Check sheet for the modelled part. Datum: model origin and axes. Units: mm. A direction names the side the tool comes from. Give positions to 0.01 mm unless a question says otherwise; leave off trailing zeros. Write each loop counter-clockwise with the first axis right and the second up, starting at its lowest first coordinate (ties: lowest second). Pieces come first, ordered by that corner, then holes. Notation, with made-up numbers: (6, -26.5) -> (33, -26.5) arc R14 cw to (33, -9.5) -> close; hole circle Ø8 at (22, 56). An arc over 180 degrees is marked (long way). Return JSON: item names as keys, results as strings.
from build123d import *

# Parameters (mm, degrees)
SKETCH1_W           = 72
SKETCH1_H           = 47
BOSS_EXTRUDE1_DEPTH = 4
SKETCH3_W           = 72
SKETCH3_H           = 47
SKETCH3_W_2         = 67
SKETCH3_H_2         = 42
BOSS_EXTRUDE3_DEPTH = 26
SKETCH5_W           = 12
SKETCH5_H           = 8
CUT_EXTRUDE1_DEPTH  = 6
FILLET2_R           = 2
FILLET3_R           = 2
SKETCH11_W          = 24
SKETCH11_H          = 20
BOSS_EXTRUDE7_DEPTH = 20
SKETCH12_W          = 20
SKETCH12_H          = 16
CUT_EXTRUDE4_DEPTH  = 20
SKETCH13_W          = 15
SKETCH13_H          = 9
CUT_EXTRUDE5_DEPTH  = 20
FILLET4_R           = 2
FILLET5_R           = 2
SKETCH14_W          = 6
SKETCH14_H          = 25
CUT_EXTRUDE6_DEPTH  = 5
FILLET6_R           = 2
SKETCH15_W          = 68
SKETCH15_H          = 6
BOSS_EXTRUDE8_DEPTH = 25
FILLET7_R           = 5
CUT_EXTRUDE7_DEPTH  = 25


with BuildPart() as part:
    # Sketch1 → Boss-Extrude1 (new body)
    with BuildSketch(Plane(origin=(0, 0, 0), x_dir=(1, 0, 0), z_dir=(0, 1, 0))):
        with Locations((25.5, 13)):
            Rectangle(SKETCH1_W, SKETCH1_H)
    extrude(amount=BOSS_EXTRUDE1_DEPTH)

    # Sketch3 → Boss-Extrude3 (add)
    with BuildSketch(Plane(origin=(0, 4, 0), x_dir=(1, 0, 0), z_dir=(0, 1, 0))):
        with Locations((25.5, 13)):
            Rectangle(SKETCH3_W, SKETCH3_H)
        with Locations((25.5, 13)):
            Rectangle(SKETCH3_W_2, SKETCH3_H_2, mode=Mode.SUBTRACT)
    extrude(amount=BOSS_EXTRUDE3_DEPTH)

    # Sketch5 → Cut-Extrude1 (cut)
    with BuildSketch(Plane(origin=(61.5, 0, 0), x_dir=(0, 0, -1), z_dir=(1, 0, 0))):
        with Locations((10, 16)):
            Rectangle(SKETCH5_W, SKETCH5_H)
    extrude(amount=-CUT_EXTRUDE1_DEPTH, mode=Mode.SUBTRACT)

    # Fillet2
    fillet2_edges = [part.edges().sort_by_distance(p)[0] for p in [
        (-10.5, 15, 10.5),
        (-10.5, 15, -36.5),
        (61.5, 15, -36.5),
        (61.5, 15, 10.5),
    ]]
    fillet(fillet2_edges, radius=FILLET2_R)

    # Fillet3
    fillet3_edges = [part.edges().sort_by_distance(p)[0] for p in [
        (60.25, 20, -4),
        (60.25, 20, -16),
    ]]
    fillet(fillet3_edges, radius=FILLET3_R)

    # Sketch11 → Boss-Extrude7 (add)
    with BuildSketch(Plane.ZY.offset(10.5)):
        with Locations((-15.5, 18)):
            Rectangle(SKETCH11_W, SKETCH11_H)
    extrude(amount=BOSS_EXTRUDE7_DEPTH)

    # Sketch12 → Cut-Extrude4 (cut)
    with BuildSketch(Plane(origin=(-8, 0, 0), x_dir=(0, 0, -1), z_dir=(1, 0, 0))):
        with Locations((15.5, 18)):
            Rectangle(SKETCH12_W, SKETCH12_H)
    extrude(amount=-CUT_EXTRUDE4_DEPTH, mode=Mode.SUBTRACT)

    # Sketch13 → Cut-Extrude5 (cut)
    with BuildSketch(Plane.ZY.offset(30.5)):
        with Locations((-15.5, 18)):
            Rectangle(SKETCH13_W, SKETCH13_H)
    extrude(amount=-CUT_EXTRUDE5_DEPTH, mode=Mode.SUBTRACT)

    # Fillet4
    fillet4_edges = [part.edges().sort_by_distance(p)[0] for p in [
        (-18, 10, -25.5),
        (-18, 10, -5.5),
        (-18, 26, -5.5),
        (-18, 26, -25.5),
    ]]
    fillet(fillet4_edges, radius=FILLET4_R)

    # Fillet5
    fillet5_edges = [part.edges().sort_by_distance(p)[0] for p in [
        (-20.5, 28, -27.5),
        (-20.5, 8, -27.5),
        (-20.5, 8, -3.5),
        (-20.5, 28, -3.5),
    ]]
    fillet(fillet5_edges, radius=FILLET5_R)

    # Sketch14 → Cut-Extrude6 (cut)
    with BuildSketch(Plane.ZY.offset(10.5)):
        with Locations((3, 24.5)):
            Rectangle(SKETCH14_W, SKETCH14_H)
    extrude(amount=-CUT_EXTRUDE6_DEPTH, mode=Mode.SUBTRACT)

    # Fillet6
    fillet6_edges = [part.edges().sort_by_distance(p)[0] for p in [
        (-9.25, 12, 0),
        (-9.25, 12, 6),
    ]]
    fillet(fillet6_edges, radius=FILLET6_R)

    # Sketch15 → Boss-Extrude8 (add)
    with BuildSketch(Plane.XY.offset(10.5)):
        with Locations((25.5, 3)):
            Rectangle(SKETCH15_W, SKETCH15_H)
    extrude(amount=BOSS_EXTRUDE8_DEPTH)

    # Fillet7
    fillet7_edges = [part.edges().sort_by_distance(p)[0] for p in [
        (-8.5, 3, 35.5),
        (59.5, 3, 35.5),
    ]]
    fillet(fillet7_edges, radius=FILLET7_R)

    # Sketch16 → Cut-Extrude7 (cut)
    with BuildSketch(Plane(origin=(0, 6, 0), x_dir=(1, 0, 0), z_dir=(0, 1, 0))):
        with BuildLine():
            Line((5.870048695, -18.078882232), (45.129951305, -18.078882232))
            ThreePointArc((45.129951305, -18.078882232), (49.279951305, -22.228882232), (45.129951305, -26.378882232))
            Line((45.129951305, -26.378882232), (5.870048695, -26.378882232))
            ThreePointArc((5.870048695, -26.378882232), (1.720048695, -22.228882232), (5.870048695, -18.078882232))
        make_face()
    extrude(amount=-CUT_EXTRUDE7_DEPTH, mode=Mode.SUBTRACT)


solid = part.part
(1) Set-up check for faces 1 (the flat face through (26, 3, 26.379)), 2 (the cylindrical face through (-18.14, 25.43, -24.9)), 3 (the flat face through (-8, 8, -17)): record each of +Z, -Z, +X, -X, +Y, -Y from which the full face is reachable in a straight line by a thin tool's end or side.
Reply:
{"face 1": "+Y, -Y", "face 2": "none", "face 3": "+Y"}
(2) Cross-section at D-D on z = -17. Enter the section's corners in (x, y).
Reply:
{"outline": "(-30.5, 8) -> (-10.5, 8) -> (-10.5, 0) -> (61.5, 0) -> (61.5, 30) -> (59, 30) -> (59, 4) -> (-8, 4) -> (-8, 10) -> (-28, 10) -> (-28, 13.5) -> (-30.5, 13.5) -> close; (-30.5, 22.5) -> (-28, 22.5) -> (-28, 26) -> (-8, 26) -> (-8, 30) -> (-10.5, 30) -> (-10.5, 28) -> (-30.5, 28) -> close"}
(3) Release check for a two-part mould opening along X. For faces 4 (the flat face through (25, 17, 8)), 5 (the flat face through (-8.5, 3, 20)), 6 (the cylindrical face through (-20.64, 27.4, -4.07)) record: pulls with the +X half, pulls with the -X half, needs draft (parallel to the pull), parting line crosses it, or undercut.
Reply:
{"face 4": "undercut", "face 5": "pulls with the -X half", "face 6": "needs draft"}
(4) Cross-section at A-A on x = 36.5. Enter the section's corners in (y, z).
Reply:
{"outline": "(0, -36.5) -> (30, -36.5) -> (30, -34) -> (4, -34) -> (4, 8) -> (30, 8) -> (30, 10.5) -> (6, 10.5) -> (6, 18.08) -> (0, 18.08) -> close; (0, 26.38) -> (6, 26.38) -> (6, 35.5) -> (0, 35.5) -> close"}
(5) Depth check by flat-ended pin: pin 1 Ø8 at (x, y) = (26.5, 14) entering from +Z; pin 2 Ø1.8 at (y, z) = (3, 18) entering from +X; pin 3 Ø1.2 at (x, y) = (61, 13.5) entering from +Z; pin 4 Ø6 at (y, z) = (15.5, 15.5) entering from +X. Enter the tip coordinate at first touch or a pass-through.
Reply:
{"pin 1": "z = 10.5", "pin 2": "x = 59.5", "pin 3": "z = 10.29", "pin 4": "through"}
(6) Thickness scan on L1, parallel to Z at x = 21.5, y = 5; L2, parallel to Z at x = 44, y = 10.75; L3, parallel to Z at x = -26, y = 13.75. Record the ranges inside material, lowest first.
Reply:
{"L1": "-36.5 to -34, 8 to 18.08, 26.38 to 35.5", "L2": "-36.5 to -34, 8 to 10.5", "L3": "-27.5 to -25.5, -5.5 to -3.5"}
(7) Cross-section at C-C on x = -17. Enter the section's corners in (y, z), then the cut area to 3 significant figures.
Reply:
{"outline": "(8, -25.5) arc R2 ccw to (10, -27.5) -> (26, -27.5) arc R2 ccw to (28, -25.5) -> (28, -5.5) arc R2 ccw to (26, -3.5) -> (10, -3.5) arc R2 ccw to (8, -5.5) -> close; hole (10, -23.5) arc R2 ccw to (12, -25.5) -> (24, -25.5) arc R2 ccw to (26, -23.5) -> (26, -7.5) arc R2 ccw to (24, -5.5) -> (12, -5.5) arc R2 ccw to (10, -7.5) -> close", "area": "160 mm^2"}
(8) Cross-section at B-B on y = 3. Enter the section's corners in (x, z).
Reply:
{"outline": "(-10.5, -34.5) arc R2 ccw to (-8.5, -36.5) -> (59.5, -36.5) arc R2 ccw to (61.5, -34.5) -> (61.5, 8.5) arc R2 ccw to (59.5, 10.5) -> (59.5, 30.5) arc R5 ccw to (54.5, 35.5) -> (-3.5, 35.5) arc R5 ccw to (-8.5, 30.5) -> (-8.5, 10.5) arc R2 ccw to (-10.5, 8.5) -> close; hole (5.87, 18.08) -> (45.13, 18.08) arc R4.15 ccw to (45.13, 26.38) -> (5.87, 26.38) arc R4.15 ccw to start"}
